```python
from build123d import *

# Parameters (mm, degrees)
SKETCH1_W                         = 99
SKETCH1_H                         = 12
BASEPLATE_DEPTH                   = 600
SKETCH2_W                         = 12
SKETCH2_H                         = 600
SIDE_RAIL_DEPTH                   = 50
SKETCH3_W                         = 24.5
SKETCH3_H                         = 600
KEEPER_RAIL_DEPTH                 = 12
SKETCH5_W                         = 99
SKETCH5_H                         = 50
LAP_JOINT_CUTOUT_DEPTH            = 12
LAP_JOINT_BOLT_HOLE_PATTERN_D     = 4.2
LAP_JOINT_BOLT_HOLE_PATTERN_DEPTH = 14
LAP_JOINT_BOLT_HOLE_PATTERN_TIP   = 1.2618073


with BuildPart() as part:
    # Sketch1 → baseplate (new body)
    with BuildSketch(Plane.XY):
        with Locations((49.5, 6)):
            Rectangle(SKETCH1_W, SKETCH1_H)
    extrude(amount=BASEPLATE_DEPTH)

    # Sketch2 → side_rail (add)
    with BuildSketch(Plane(origin=(0, 12, 0), x_dir=(1, 0, 0), z_dir=(0, 1, 0))):
        with Locations((6, -300)):
            Rectangle(SKETCH2_W, SKETCH2_H)
    side_rail = extrude(amount=SIDE_RAIL_DEPTH)

    # Sketch3 → keeper rail (add)
    with BuildSketch(Plane(origin=(0, 62, 0), x_dir=(1, 0, 0), z_dir=(0, 1, 0))):
        with Locations((12.25, -300)):
            Rectangle(SKETCH3_W, SKETCH3_H)
    keeper_rail = extrude(amount=KEEPER_RAIL_DEPTH)

    # mirror rails: side_rail, keeper rail across plane
    add(side_rail.mirror(Plane.ZY.offset(-49.5)))
    add(keeper_rail.mirror(Plane.ZY.offset(-49.5)))

    # Sketch5 → lap joint cutout (cut)
    with BuildSketch(Plane.XZ):
        with Locations((49.5, 25)):
            Rectangle(SKETCH5_W, SKETCH5_H)
    extrude(amount=-LAP_JOINT_CUTOUT_DEPTH, mode=Mode.SUBTRACT)

    # lap joint bolt hole pattern
    with Locations(Plane(origin=(0, 12, 0), x_dir=(-1, 0, 0), z_dir=(0, -1, 0))):
        with Locations((-93, -10), (-6, -40), (-93, -40), (-6, -10)):
            Hole(LAP_JOINT_BOLT_HOLE_PATTERN_D / 2, depth=LAP_JOINT_BOLT_HOLE_PATTERN_DEPTH)
            with Locations((0, 0, -(LAP_JOINT_BOLT_HOLE_PATTERN_DEPTH + LAP_JOINT_BOLT_HOLE_PATTERN_TIP / 2))):  # 118° drill point
                Cone(0, LAP_JOINT_BOLT_HOLE_PATTERN_D / 2, LAP_JOINT_BOLT_HOLE_PATTERN_TIP, mode=Mode.SUBTRACT)


solid = part.part
```
The model under review builds one solid part; all positions refer to its coordinate system, in mm. A direction names the side the tool comes from. Round coordinates to 2 decimals unless told otherwise and drop trailing zeros. Loops run counter-clockwise (first coordinate to the right, second up) from the corner with the lowest first, then second, coordinate; pieces in that order, holes last. Notation, with made-up numbers: M 4.5,56 L 12.5,56 A24 cw 12.5,83 Z; hole C -33,55 d5. An arc over 180 degrees is marked long. Write item = value, one per line.
Item 1: Take a section at A-A on x = 18. Write out the cut boundary in (y, z).
Return value:
outline = M 0,50 L 12,50 L 12,600 L 0,600 Z; M 62,0 L 74,0 L 74,600 L 62,600 Z
Item 2: Take a section at C-C on z = 430.5. Write out the cut boundary in (x, y).
Return value:
outline = M 0,0 L 99,0 L 99,74 L 74.5,74 L 74.5,62 L 87,62 L 87,12 L 12,12 L 12,62 L 24.5,62 L 24.5,74 L 0,74 Z
Item 3: Insertion check: P1, Ø6, axis at x = 91, z = 22, coming from the -Y side; P2, Ø1.5, axis at x = 50, z = 466, coming from the +Y side; P3, Ø3.5, axis at x = 73.5, y = 3.5, coming from the -Z side. Each pin has a flat end and moves straight along its axis. Give the tip position at first contact, or say it passes through.
Return value:
P1 = 12
P2 = 12
P3 = 50
Item 4: Take a section at D-D on x = 64.5. Write out the cut boundary in (y, z).
Return value:
outline = M 0,50 L 12,50 L 12,600 L 0,600 Z
Item 5: For line 1 (X direction, y = 18.5, z = 40); line 2 (Z direction, x = 93, y = 22.5); line 3 (Y direction, x = 21, z = 355), list the stretches that pass through material, from the lowest coordinate up. Write a range as [from, to].
Return value:
line_1 = [0, 3.9], [8.1, 12], [87, 90.9], [95.1, 99]
line_2 = [0, 7.9], [12.1, 37.9], [42.1, 600]
line_3 = [0, 12], [62, 74]
Item 6: Take a section at B-B on y = 20. Write out the cut boundary in (x, z), then the cut area to 3 significant figures.
Return value:
outline = M 0,0 L 12,0 L 12,600 L 0,600 Z; M 87,0 L 99,0 L 99,600 L 87,600 Z; hole C 6,10 d4.2; hole C 6,40 d4.2; hole C 93,10 d4.2; hole C 93,40 d4.2
area = 14,300 mm2
Item 7: Machinability: for faces 1 (the flat face through (74.5, 68, 304)), 2 (the flat face through (50.2, 11.8, 600)), 3 (the flat face through (49, 6, 50)), 4 (the flat face through (49, 12, 321)), 5 (the flat face through (87, 74, 296)), which of the approach directions +Z, -Z, +X, -X, +Y, -Y give a long, thin tool a straight path to every point of the face, cutting with its end or side? Answer none if there is none.
Return value:
face_1 = +Z, -Z, +Y
face_2 = +Z, +X, -X, +Y, -Y
face_3 = -Z, +X, -X, -Y
face_4 = +Z, -Z
face_5 = +Z, -Z, +X, -X, +Y
Item 8: The part is to be moulded in two halves that separate along X. For faces 6 (the flat face through (99, 36, 304)), 7 (the flat face through (0, 36, 304)), 8 (the flat face through (81, 62, 296)), 9 (the flat face through (12, 74, 296)), say which applies: released by +X, released by -X, zero draft, split by the parting line, or undercut.
Return value:
face_6 = released by +X
face_7 = released by -X
face_8 = undercut
face_9 = zero draft
